from build123d import *

# Parameters (mm, degrees)
BASPROSKE_W         = 30
BASPROSKE_H         = 55
TOOTHCUT_DEPTH      = 84.366660003
TEETHCUTS_COUNT     = 20
BORSKE_R            = 2.5
BORE_DEPTH          = 50.0000508
EXTRUDE_START       = -30
EXTRUDE_1_DEPTH     = 30
SKETCH_7_R          = 2.5
CUT_EXTRUDE_1_DEPTH = 160.570441323


with BuildPart() as part:
    # BasProSke → Base-Revolve (revolve)
    with BuildSketch(Plane(origin=(0, 0, 0), x_dir=(1, 0, 0), z_dir=(0, 1, 0)), mode=Mode.PRIVATE) as base_revolve_sk:
        with Locations((15, 27.5)):
            Rectangle(BASPROSKE_W, BASPROSKE_H)
    revolve(base_revolve_sk.sketch.rotate(Axis((-10, 0, 0), (1, 0, 0)), 180), axis=Axis((-10, 0, 0), (1, 0, 0)))

    # TooCutSke → ToothCut (cut, through all)
    with BuildSketch(Plane(origin=(0, 0, 0), x_dir=(0, 0, -1), z_dir=(1, 0, 0))):
        with BuildLine():
            ThreePointArc((2.464838288, 43.679509764), (0, 43.749), (-2.464838288, 43.679509764))
            ThreePointArc((-2.464838288, 43.679509764), (-4.057398861, 49.476814676), (-7.300899231, 54.538899105))
            ThreePointArc((-7.300899231, 54.538899105), (0, 55.0254), (7.300899231, 54.538899105))
            ThreePointArc((7.300899231, 54.538899105), (4.057398861, 49.476814676), (2.464838288, 43.679509764))
        make_face()
    toothcut = extrude(amount=TOOTHCUT_DEPTH, mode=Mode.SUBTRACT)

    # TeethCuts: ToothCut ×20 about axis
    teethcuts_axis = Axis((0, 0, 0), (1, 0, 0))
    for i in range(1, TEETHCUTS_COUNT):
        add(toothcut.rotate(teethcuts_axis, i * 360 / TEETHCUTS_COUNT), mode=Mode.SUBTRACT)

    # BorSke → Bore (cut, symmetric)
    with BuildSketch(Plane(origin=(0, 0, 0), x_dir=(0, 0, -1), z_dir=(1, 0, 0))):
        with Locations(Location((0, 0, 0), (0, 0, 180))):
            Circle(BORSKE_R)
    extrude(amount=BORE_DEPTH, both=True, mode=Mode.SUBTRACT)

    # 草图6 → 凸台-拉伸1 (add)
    with BuildSketch(Plane(origin=(30, 0, 0), x_dir=(0, 0, -1), z_dir=(1, 0, 0)).offset(EXTRUDE_START)):
        with BuildLine():
            Line((-11.153510308, -42.303359309), (-11.153510308, -142.303359309))
            Line((-11.153510308, -142.303359309), (11.153510308, -142.303359309))
            Line((11.153510308, -142.303359309), (11.153510308, -42.303359309))
            ThreePointArc((11.153510308, -42.303359309), (0, -43.749), (-11.153510308, -42.303359309))
        make_face()
    extrude(amount=EXTRUDE_1_DEPTH)

    # 草图7 → 切除-拉伸1 (cut, through all)
    with BuildSketch(Plane.XY.offset(11.153510308)):
        with Locations((15, -131.019533407)):
            Circle(SKETCH_7_R)
    extrude(amount=-CUT_EXTRUDE_1_DEPTH, mode=Mode.SUBTRACT)


solid = part.part
The listing builds one solid part. Answer for the finished solid, in the listing's coordinates (mm). A direction names the side the tool comes from. Round coordinates to 2 decimals unless told otherwise and drop trailing zeros. Write each loop counter-clockwise with the first axis right and the second up, starting at its lowest first coordinate (ties: lowest second). Pieces come first, ordered by that corner, then holes. Notation, with made-up numbers: M 56.25,44 L 100.25,44 A34 cw 100.25,77 Z; hole C 31.25,76.5 d6. An arc over 180 degrees is marked long. Write each question's results on one line, items separated by ' | '. Start each with the question number.
Item 1: A cutting plane is placed at B-B on z = 0. Write down the section's boundary in (x, y).
Item 2: For faces 5 (the face through (14.79, -11.423, 48.378)), 6 (the face through (14.79, 37.677, -32.424)), 7 (the face through (15, -96, 11.154)), 8 (the face through (14.79, -4.02, 49.39)), determine the directions among +Z, -Z, +X, -X, +Y, -Y from which every point of the face is accessible in a straight line to the end or side of a thin tool.
Item 3: A cutting plane is placed at C-C on x = 15. State how many separate pieces and enclosed holes the cut face has, and give its area (3 significant figures).
Item 4: A cutting plane is placed at D-D on y = -46. Write down the section's boundary in (x, z), and give its area (3 significant figures).
Item 5: Straight lines are drawn through the part: L1, parallel to Y at x = 19.5, z = 0; L2, parallel to Y at x = 9, z = 34; L3, parallel to Z at x = 22.25, y = -36. For each, find the intervals that lie inside material, in ascending order. Write a range as [from, to].
Item 6: For a pull along Y with two mould halves and no side action, classify faces 1 (the face through (14.79, 37.593, 32.278)), 2 (the face through (14.79, -4.086, -49.54)), 3 (the face through (15, -142.303, 0)), 4 (the face through (14.79, -13.552, -41.597)) as pulls with the +Y half, pulls with the -Y half, needs draft (parallel to the pull), parting line crosses it, or undercut.
Item 7: Flat-ended cylindrical pins translate along their axes: pin 1 Ø1 at (x, z) = (5.5, -23) entering from +Y; pin 2 Ø5 at (x, z) = (23.5, 29) entering from -Y; pin 3 Ø4 at (x, y) = (14.5, 29) entering from -Z. Find the tip coordinate at first contact, or state that the pin passes through.
Item 8: A cutting plane is placed at A-A on y = 0. Write down the section's boundary in (x, z).
Check sheet entries:
1) outline: M 0,-142.3 L 30,-142.3 L 30,-2.5 L 0,-2.5 Z; M 0,2.5 L 30,2.5 L 30,43.75 L 0,43.75 Z; hole C 15,-131.02 d5
2) face 5: +X, -X | face 6: +X, -X, +Y | face 7: +Z, +X, -X, -Y | face 8: +Z, +X, -X
3) separate pieces: 2 | enclosed holes: 1 | area: 9,510 mm²
4) outline: M 0,-26.23 L 30,-26.23 L 30,-19.33 L 0,-19.33 Z; M 0,-11.54 L 30,-11.54 L 30,11.54 L 0,11.54 Z; M 0,19.33 L 30,19.33 L 30,26.23 L 0,26.23 Z | area: 1,110 mm²
5) L1: [-142.3, -2.5], [2.5, 43.75] | L2: [-38.49, -27.77], [-27.53, 27.53], [27.77, 38.49] | L3: [-39.28, -29.95], [-24.86, 24.86], [29.95, 39.28]
6) face 1: pulls with the +Y half | face 2: undercut | face 3: pulls with the -Y half | face 4: undercut
7) pin 1: y = 49.43 | pin 2: y = -37.11 | pin 3: z = -36.78
8) outline: M 0,-43.75 L 30,-43.75 L 30,-2.5 L 0,-2.5 Z; M 0,2.5 L 30,2.5 L 30,43.75 L 0,43.75 Z
